```python
from build123d import *

# Parameters (mm, degrees)
F0_W     = 279.4
F0_H     = 482.6
F1_DEPTH = 381
F2_R     = 5
F3_T     = -2.54


# Not quite as in the source:
# - a shell that OpenCascade refuses in one call is made with other operations: the cavity is built on its own and cut out


with BuildPart() as f1:
    # F0 (on Front) → F1 (new body)
    with BuildSketch(Plane.XZ):
        Rectangle(F0_W, F0_H)
    extrude(amount=F1_DEPTH)

    # F2
    f2_edges = [f1.edges().sort_by_distance(p)[0] for p in [
        (139.7, -190.5, 241.3),
        (-139.7, -190.5, 241.3),
        (139.7, -190.5, -241.3),
        (139.7, 0, 0),
        (0, 0, 241.3),
        (-139.7, -381, 0),
        (0, -381, -241.3),
        (0, -381, 241.3),
    ]]
    fillet(f2_edges, radius=F2_R)

    # F3: a shell. OpenCascade refuses it in one call, so the cavity is built on its own and cut out:
    # the body offset inwards by the wall thickness, plus a prism from it out through each open face.
    f3_core = offset(f1.part, amount=F3_T, mode=Mode.PRIVATE)
    f3_exits = [f3_core.faces().sort_by_distance(p)[0] for p in [
        (1.23, -378.46, 0),
    ]]
    add(f3_core, mode=Mode.SUBTRACT)
    extrude(f3_exits, amount=-F3_T, mode=Mode.SUBTRACT)


solid = f1.part
```
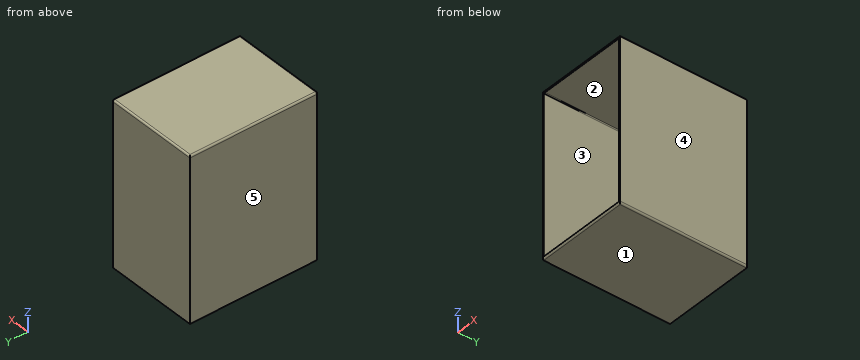
Part model, mm, in its own coordinate system. Face numbers are marked on the shaded views. A direction names the side the tool comes from. Round coordinates to 2 decimals unless told otherwise and drop trailing zeros. Write each loop counter-clockwise with the first axis right and the second up, starting at its lowest first coordinate (ties: lowest second). Pieces come first, ordered by that corner, then holes. Notation, with made-up numbers: M 35.5,39.5 L 55.5,39.5 A16 cw 55.5,68.5 Z; hole C 46.25,45.5 d3. An arc over 180 degrees is marked long. One line per question, with ' | ' between items.
(1) 3-axis set-ups, long thin cutter, end or side, ignore diameter. For the marked faces 1 and 2: which of +Z, -Z, +X, -X, +Y, -Y reach the whole face in a straight line?
Answer key:
face 1: -Z, +X, -X, +Y, -Y | face 2: none
(2) Two-plate mould, pull along X, no slides. Class the marked faces 3, 4 and 5: released by +X, released by -X, zero draft, split by the parting line, or undercut.
Answer key:
face 3: undercut | face 4: released by +X | face 5: released by -X
(3) Saw through at A-A on y = -279.5. Write the cut outline in (x, z).
Answer key:
outline: M -139.7,-241.3 L 134.7,-241.3 A5 ccw 139.7,-236.3 L 139.7,236.3 A5 ccw 134.7,241.3 L -134.7,241.3 A5 ccw -139.7,236.3 Z; hole M -137.16,-238.76 L 134.7,-238.76 A2.46 ccw 137.16,-236.3 L 137.16,236.3 A2.46 ccw 134.7,238.76 L -134.7,238.76 A2.46 ccw -137.16,236.3 Z
(4) Saw through at B-B on x = 73.5. Write the cut outline in (y, z), then the cut area to 3 significant figures.
Answer key:
outline: M -381,-236.3 A5 ccw -376,-241.3 L 0,-241.3 L 0,236.3 A5 ccw -5,241.3 L -376,241.3 A5 ccw -381,236.3 L -378.46,236.3 A2.46 cw -376,238.76 L -5,238.76 A2.46 cw -2.54,236.3 L -2.54,-238.76 L -376,-238.76 A2.46 cw -378.46,-236.3 Z | area: 3,150 mm^2
(5) Saw through at C-C on z = 142. Write the cut outline in (x, y).
Answer key:
outline: M -139.7,-376 A5 ccw -134.7,-381 L -134.7,-378.46 A2.46 cw -137.16,-376 L -137.16,-2.54 L 134.7,-2.54 A2.46 cw 137.16,-5 L 137.16,-381 L 139.7,-381 L 139.7,-5 A5 ccw 134.7,0 L -139.7,0 Z
(6) Pin check, flat tips, straight feed: pin 1 (2 mm diameter, centred on x = -13, y = -380, fed in from +Z); pin 2 (2 mm diameter, centred on x = 62.5, y = -380, fed in from -Z); pin 3 (2 mm diameter, centred on x = -7, z = 154, fed in from +Y). Stop position of each tip, or through.
Answer key:
pin 1: stops at z = 240.3 | pin 2: stops at z = -240.3 | pin 3: stops at y = 0
(7) Probe line 1 along Z through (x, y) = (-5, -149); line 2 along X through (y, z) = (-313.5, -70.5); line 3 along Y through (x, z) = (99, 98). List the from-to ranges inside material, lowest first.
Answer key:
line 1: z = -241.3 to -238.76, 238.76 to 241.3 | line 2: x = -139.7 to -137.16, 137.16 to 139.7 | line 3: y = -2.54 to 0
